Part model, mm, in its own coordinate system. Face numbers are marked on the shaded views. Round coordinates to 2 decimals unless told otherwise and drop trailing zeros. Loops run counter-clockwise (first coordinate to the right, second up) from the corner with the lowest first, then second, coordinate; pieces in that order, holes last.
1) Drop flat-ended pins along their axis: P1, Ø5, axis at y = 0.5, z = 3.5, coming from the -X side; P2, Ø4, axis at x = 1.5, z = 6, coming from the +Y side; P3, Ø8, axis at x = 0, y = 0.5, coming from the -Z side; P4, Ø7.5, axis at x = 0, y = 0, coming from the -Z side. Give the stop position or say it passes through.
2) Band-saw the part on D-D, the plane x = 6.75. Write the cut outline in (y, z), then the cut area to 3 significant figures.
3) Mould opens along Y. For the marked faces 1, 2 and 3 say: +Y half, -Y half, draft (parallel to the pull), parting line (faces both ways), or undercut.
4) Probe line 1 (Y direction, x = 0, z = 6.5); line 2 (Z direction, x = 5.75, y = -4.25); line 3 (Y direction, x = -2.5, z = 3.5). List the from-to ranges inside material, lowest first.
5) Band-saw the part on A-A, the plane y = 0. Write the cut outline in (x, z).
6) Band-saw the part on C-C, the plane z = 7.5. Write the cut outline in (x, y), then the cut area to 3 significant figures.
Autodesk Inventor part; units mm, degrees
ref_plane "YZ Plane" through (0, 0, 0) normal (1, 0, 0) x (0, 1, 0)
ref_plane "XZ Plane" through (0, 0, 0) normal (0, 1, 0) x (-1, 0, 0)
ref_plane "XY Plane" through (0, 0, 0) normal (0, 0, 1) x (1, 0, 0)
sketch "Sketch1" plane through (0, 0, 0) normal (0, 0, 1) x (1, 0, 0)
  point P0 (0, 0)
sketch "Sketch2" plane through (0, 0, 0) normal (0, 0, 1) x (1, 0, 0)
  circle A0 centre (0, 0) radius 6.35
  circle A1 centre (0, 0) radius 4.1783
  dimension "d0" = 8.3566
  dimension "d1" = 12.7
extrude "Extrusion1" add sketch "Sketch2" along normal blind 7.747
sketch "Sketch3" plane through (0, 0, 7.747) normal (0, 0, 1) x (1, 0, 0)
  circle A0 centre (0, 0) radius 4.1783
  circle A1 centre (0, 0) radius 8.0645
  dimension "d4" = 16.129
extrude "Extrusion2" add sketch "Sketch3" along normal blind 1.27
chamfer "Chamfer1" distance 0.508 angle 45 3 edges at (-4.1783, 0, 0) (-6.35, 0, 0) (-4.1783, 0, 9.017)
properties part number "robotics"
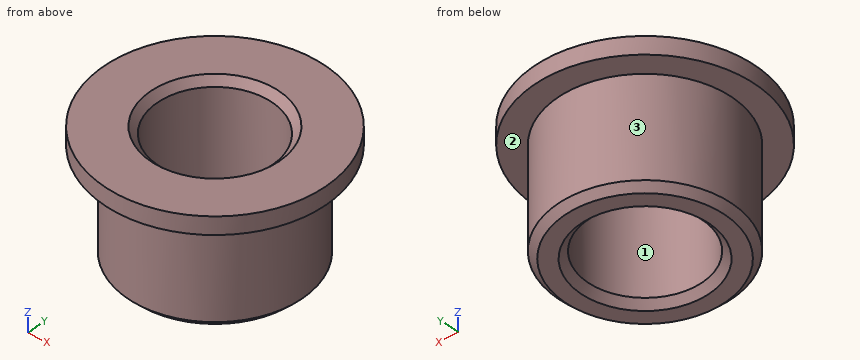
Reported:
1. P1: stops at x = -6.35
1. P2: stops at y = 8.05
1. P3: stops at z = 0.19
1. P4: passes through
2. outline: (-4.41, 7.75) - (4.41, 7.75) - (4.41, 9.02) - (-4.41, 9.02) - close
2. area: 11.2 mm2
3. face 1: undercut
3. face 2: draft
3. face 3: parting line
4. line 1: y = -6.35 to -4.18, 4.18 to 6.35
4. line 2: z = 7.75 to 9.02
4. line 3: y = -5.84 to -3.35, 3.35 to 5.84
5. outline: (-8.06, 7.75) - (-6.35, 7.75) - (-6.35, 0.51) - (-5.84, 0) - (-4.69, 0) - (-4.18, 0.51) - (-4.18, 8.51) - (-4.69, 9.02) - (-8.06, 9.02) - close; (4.18, 0.51) - (4.69, 0) - (5.84, 0) - (6.35, 0.51) - (6.35, 7.75) - (8.06, 7.75) - (8.06, 9.02) - (4.69, 9.02) - (4.18, 8.51) - close
6. outline: circle Ø12.7 at (0, 0); hole circle Ø8.36 at (0, 0)
6. area: 71.8 mm2
